```python
from build123d import *

# Parameters (mm, degrees)
SKETCH1_R                       = 8.610000052
SKETCH1_R_2                     = 4.999999906
BOSS_EXTRUDE1_DEPTH             = 54.356
SKETCH2_W                       = 1.89865
SKETCH2_H                       = 8.610000052
F_10_24_TAPPED_HOLE1_AT_2_COUNT = 2
F_10_24_TAPPED_HOLE1_AT_2_PITCH = 28.956
SKETCH8_W                       = 2.45745
SKETCH8_H                       = 8.610000052


with BuildPart() as part:
    # Sketch1 → Boss-Extrude1 (new body)
    with BuildSketch(Plane.XY):
        Circle(SKETCH1_R)
        Circle(SKETCH1_R_2, mode=Mode.SUBTRACT)
    extrude(amount=BOSS_EXTRUDE1_DEPTH)

    # Sketch2 → #10-24 Tapped Hole1 (revolve, cut)
    with BuildSketch(Plane(origin=(0, 0, 12.7), x_dir=(0, 0, -1), z_dir=(1, 0, 0))):
        with Locations((0.949325, 4.305000026)):
            Rectangle(SKETCH2_W, SKETCH2_H)
    f_10_24_tapped_hole1 = revolve(axis=Axis((0, -6.35, 12.7), (0, 1, 0)), mode=Mode.SUBTRACT)

    # #10-24 Tapped Hole1 at 2: #10-24 Tapped Hole1 ×2
    with Locations(*[(0, 0, i * F_10_24_TAPPED_HOLE1_AT_2_PITCH) for i in range(1, F_10_24_TAPPED_HOLE1_AT_2_COUNT)]):
        add(f_10_24_tapped_hole1, mode=Mode.SUBTRACT)

    # Sketch8 → #10 (0.1935) Diameter Hole3 (revolve, cut)
    with BuildSketch(Plane(origin=(0, 0, 41.656), x_dir=(0, 0, 1), z_dir=(1, 0, 0))):
        with Locations((1.228725, 4.305000026)):
            Rectangle(SKETCH8_W, SKETCH8_H)
    revolve(axis=Axis((0, 6.35, 41.656), (0, -1, 0)), mode=Mode.SUBTRACT)


solid = part.part
```
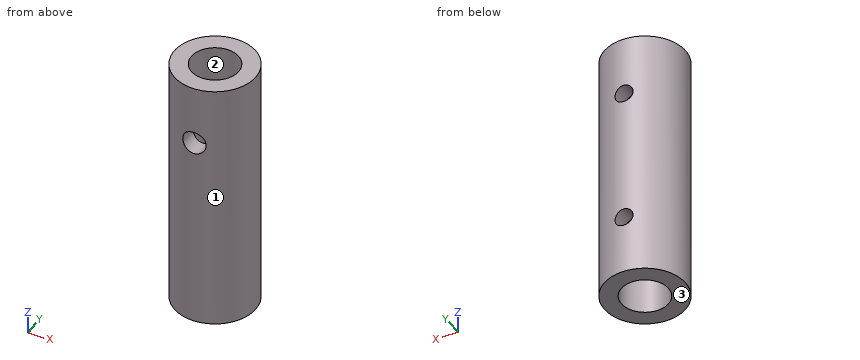
Input: part model. Units: mm. Frame: model coordinates. Face numbers are marked on the shaded views. Coordinates: 2 decimals unless noted, no trailing zeros. Loops run counter-clockwise (first coordinate to the right, second up) from the corner with the lowest first, then second, coordinate; pieces in that order, holes last. Notation, with made-up numbers: M -30.75,-34 L -17.75,-34 A23 cw -17.75,-6 Z; hole C -34,-2.75 d1. An arc over 180 degrees is marked long. One line per item, written item: value.
(1) Section C-C (z = 15.5). Output: boundary loops of the cut face in (x, y).
Filled in:
outline: C 0,0 d17.22; hole C 0,0 d10
(2) Pin query (flat end, axial travel): pin 1 (2 mm diameter, centred on x = -2, y = 0.5, fed in from +Z); pin 2 (8 mm diameter, centred on y = -4.5, z = 40, fed in from +X); pin 3 (8 mm diameter, centred on x = 6.5, z = 30.5, fed in from -Y); pin 4 (2.5 mm diameter, centred on x = 0, z = 12.7, fed in from +Y). Return the tip coordinate at first contact, or that it passes through.
Filled in:
pin 1: through
pin 2: x = 8.6
pin 3: y = -8.24
pin 4: y = -4.84
(3) Section D-D (y = -5.75). Output: boundary loops of the cut face in (x, z).
Filled in:
outline: M -6.41,0 L 6.41,0 L 6.41,54.36 L -6.41,54.36 Z; hole C 0,41.66 d4.91
(4) Pull-direction query (X, two-part tool) for the marked faces 1, 2 and 3; classes: +X half, -X half, draft (parallel to the pull), parting line (faces both ways), or undercut.
Filled in:
face 1: parting line
face 2: undercut
face 3: draft
(5) Section B-B (x = 0). Output: boundary loops of the cut face in (y, z).
Filled in:
outline: M -8.61,0 L -5,0 L -5,39.2 L -8.61,39.2 Z; M -8.61,44.11 L -5,44.11 L -5,54.36 L -8.61,54.36 Z; M 5,0 L 8.61,0 L 8.61,10.8 L 5,10.8 Z; M 5,14.6 L 8.61,14.6 L 8.61,39.76 L 5,39.76 Z; M 5,43.55 L 8.61,43.55 L 8.61,54.36 L 5,54.36 Z
(6) Line query: line 1 along Z through (x, y) = (0, 5.6); line 2 along Z through (x, y) = (0, -6); line 3 along Y through (x, z) = (0, 25.5). Output: solid intervals per line, ascending. Write a range as from..to.
Filled in:
line 1: 0..10.8, 14.6..39.76, 43.55..54.36
line 2: 0..39.2, 44.11..54.36
line 3: -8.61..-5, 5..8.61
(7) Section A-A (y = 0). Output: boundary loops of the cut face in (x, z), and give its area (3 significant figures).
Filled in:
outline: M -8.61,0 L -5,0 L -5,54.36 L -8.61,54.36 Z; M 5,0 L 8.61,0 L 8.61,54.36 L 5,54.36 Z
area: 392 mm^2
